Geometry check sheet. Reference: the model listing, model coordinates, mm. Round coordinates to 2 decimals unless told otherwise and drop trailing zeros. Write each loop counter-clockwise with the first axis right and the second up, starting at its lowest first coordinate (ties: lowest second). Pieces come first, ordered by that corner, then holes.
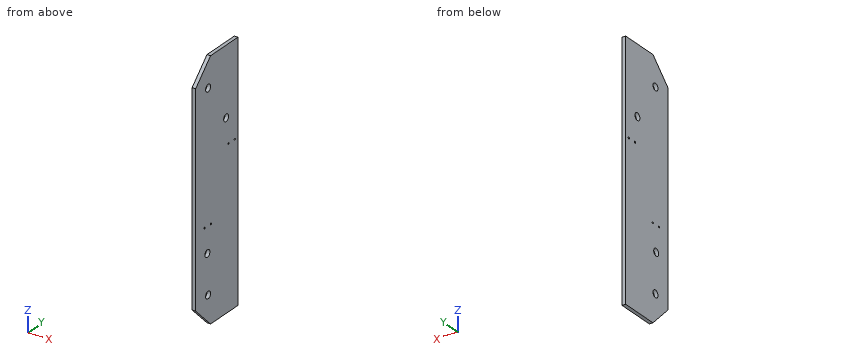
Autodesk Inventor part; units mm, degrees
ref_plane "YZ Plane" through (0, 0, 0) normal (1, 0, 0) x (0, 1, 0)
ref_plane "XZ Plane" through (0, 0, 0) normal (0, 1, 0) x (-1, 0, 0)
ref_plane "XY Plane" through (0, 0, 0) normal (0, 0, 1) x (1, 0, 0)
sketch "Sketch1" plane through (0, 0, 0) normal (1, 0, 0) x (0, 1, 0)
  line L0 (0, 0) -> (107.95, 0)
  line L1 (107.95, 0) -> (107.95, -444.5)
  line L2 (107.95, -444.5) -> (0, -444.5)
  line L3 (0, -444.5) -> (0, 0)
  circle A0 centre (31.75, -50.8) radius 6.3627
  circle A1 centre (31.75, -393.7) radius 6.3627
  circle A2 centre (92.6338, -165.5318) radius 1.5875
  circle A3 centre (76.6318, -165.5318) radius 1.5875
  circle A4 centre (15.3162, -278.9682) radius 1.5875
  circle A5 centre (31.3182, -278.9682) radius 1.5875
  dimension "d0" = 107.95
  dimension "d1" = 444.5
  dimension "d2" = 12.7254
  dimension "d3" = 31.75
  dimension "d4" = 50.8
  dimension "d5" = 50.8
  dimension "d22" = 165.5318
  dimension "d23" = 3.175
  dimension "d24" = 15.3162
  dimension "d25" = 3.175
  dimension "d26" = 16.002
  dimension "d27" = 165.5318
  dimension "d28" = 3.175
  dimension "d29" = 15.3162
  dimension "d30" = 165.5318
  dimension "d31" = 3.175
  dimension "d32" = 16.002
  dimension "d33" = 165.5318
extrude "Extrusion1" add sketch "Sketch1" along normal blind 6.35 contours L0 L1 L2 L3 | A2 | A3 | A4 | A5
chamfer "Chamfer1" distance 38.1 angle 45 1 edges at (3.175, 0, 0)
chamfer "Chamfer2" distance 38.1 angle 45 1 edges at (3.175, 0, -444.5)
sketch "Sketch2" plane through (6.35, 0, 0) normal (1, 0, 0) x (0, 0, -1)
  line L0 (444.5, 38.1) -> (406.4, 0)
  line L1 (444.5, 38.1) -> (444.5, 107.95)
  line L2 (444.5, 107.95) -> (0, 107.95)
  line L3 (0, 107.95) -> (0, 38.1)
  line L4 (38.1, 0) -> (0, 38.1)
  line L5 (38.1, 0) -> (406.4, 0)
  circle A0 centre (393.7, 31.75) radius 6.3627
  circle A1 centre (50.8, 31.75) radius 6.3627
  circle A2 centre (120.4214, 77.9526) radius 6.3627
  circle A3 centre (324.0786, 29.9974) radius 6.3627
  point P0 (0, 0)
  dimension "d14" = 12.7254
  dimension "d15" = 120.4214
  dimension "d16" = 29.9974
  dimension "d17" = 12.7254
  dimension "d18" = 29.9974
  dimension "d19" = 120.4214
extrude "Extrusion2" cut sketch "Sketch2" against normal blind 25.4 contours A2 | A3
sketch "Sketch3" plane through (6.35, 0, 0) normal (1, 0, 0) x (0, 0, -1)
  circle A0 centre (120.4214, 77.9526) radius 6.3627
  circle A1 centre (324.0786, 29.9974) radius 6.3627
  line L0 (444.5, 38.1) -> (406.4, 0)
  line L1 (444.5, 38.1) -> (444.5, 107.95)
  line L2 (444.5, 107.95) -> (0, 107.95)
  line L3 (0, 107.95) -> (0, 38.1)
  line L4 (38.1, 0) -> (0, 38.1)
  line L5 (38.1, 0) -> (406.4, 0)
  circle A2 centre (393.7, 31.75) radius 6.3627
  circle A3 centre (50.8, 31.75) radius 6.3627
  circle A4 centre (165.5318, 99.949) radius 1.5875
  circle A5 centre (165.5318, 83.947) radius 1.5875
  circle A6 centre (278.9682, 22.86) radius 1.5875
  circle A7 centre (278.9682, 38.862) radius 1.5875
  point P0 (0, 0)
  dimension "d34" = 3.175
  dimension "d35" = 165.5318
  dimension "d36" = 8.001
  dimension "d37" = 3.175
  dimension "d38" = 16.002
  dimension "d39" = 3.175
  dimension "d40" = 3.175
  dimension "d41" = 22.86
  dimension "d42" = 16.002
  dimension "d43" = 165.5318
extrude "Extrusion3" cut sketch "Sketch3" against normal blind 25.4 contours A4 | A5 | A6 | A7
properties part number "DriveTrain3.0"
1. Section check B-B (x = 5.25). State how many separate pieces and enclosed holes the cut face has, plus the area to 3 significant figures.
2. Section check A-A (z = -393.7). Record the cut outline in (x, y), plus the area to 3 significant figures.
3. Depth check by flat-ended pin: pin 1 Ø11.5 at (y, z) = (31.75, -393.7) entering from +X; pin 2 Ø5 at (y, z) = (22.86, -278.97) entering from +X; pin 3 Ø1.5 at (x, y) = (2.5, 14) entering from -Z. Enter the tip coordinate at first touch or a pass-through.
4. Scan lines: line 1 along Y through (x, z) = (2.5, -121); line 2 along Y through (x, z) = (2, -166); line 3 along Y through (x, z) = (1.5, -50.5). Record each from-to range of solid material in increasing order.
5. Section check C-C (y = 11.5). Record the cut outline in (x, z).
Results below:
1. separate pieces: 1
1. enclosed holes: 8
1. area: 46,000 mm2
2. outline: (0, 0) - (6.35, 0) - (6.35, 25.39) - (0, 25.39) - close; (0, 38.11) - (6.35, 38.11) - (6.35, 107.95) - (0, 107.95) - close
2. area: 605 mm2
3. pin 1: passes through
3. pin 2: stops at x = 6.35
3. pin 3: stops at z = -421.15
4. line 1: y = 0 to 71.62, 84.29 to 107.95
4. line 2: y = 0 to 82.43, 85.46 to 98.43, 101.47 to 107.95
4. line 3: y = 0 to 25.39, 38.11 to 107.95
5. outline: (0, -417.9) - (6.35, -417.9) - (6.35, -26.6) - (0, -26.6) - close
